Can you work these out from the model? Positions are in its coordinate system, mm. Face numbers are marked on the shaded views. A direction names the side the tool comes from. Round coordinates to 2 decimals unless told otherwise and drop trailing zeros. Loops run counter-clockwise (first coordinate to the right, second up) from the corner with the lowest first, then second, coordinate; pieces in that order, holes last.
(1) If I drill on line 1 along Y through (x, z) = (-0.25, -1.75); line 2 along Y through (x, z) = (0, 3.05); line 3 along Y through (x, z) = (0.25, 4.25), over which ranges is the centre line in solid material (lowest first)?
(2) I want a section at A-A on z = 3.75. Write out the boundary of the cut face in (x, y), plus the area to 3 significant figures.
(3) Will these pins go through, and if not, where does the flat tip stop? pin 1 Ø2 at (x, z) = (3, 0) entering from -Y; pin 2 Ø1 at (y, z) = (3, 1) entering from +X; pin 3 Ø3.5 at (x, y) = (-0.5, 2) entering from -Z.
(4) Thinking about a two-plate mould opening in Y: for the marked faces 3 and 4, which applies, released by +Y, released by -Y, zero draft, split by the parting line, or undercut?
(5) I want a section at B-B on z = 0.5. Write out the boundary of the cut face in (x, y), plus the area to 3 significant figures.
(6) Which directions (+Z, -Z, +X, -X, +Y, -Y) give clear straight access to the entire face, cutting with the end or side of a thin tool? Please do the marked faces 1 and 2.
from build123d import *

# Parameters (mm, degrees)
SKETCH1_R           = 8.5
BOSS_EXTRUDE1_DEPTH = 4.4
SKETCH3_R           = 5.8
CUT_EXTRUDE1_DEPTH  = 4
BOSS_EXTRUDE3_START = 3
SKETCH4_R           = 8.5
SKETCH4_R_2         = 7.5
BOSS_EXTRUDE3_DEPTH = 3
BOSS_EXTRUDE4_DEPTH = 0.6


with BuildPart() as part:
    # Sketch1 → Boss-Extrude1 (new body)
    with BuildSketch(Plane.XY):
        Circle(SKETCH1_R)
    extrude(amount=BOSS_EXTRUDE1_DEPTH)

    # Sketch3 → Cut-Extrude1 (cut)
    with BuildSketch(Plane(origin=(0, 0, 0), x_dir=(-1, 0, 0), z_dir=(0, 0, -1))):
        Circle(SKETCH3_R)
    extrude(amount=-CUT_EXTRUDE1_DEPTH, mode=Mode.SUBTRACT)

    # Sketch4 → Boss-Extrude3 (add)
    with BuildSketch(Plane(origin=(0, 0, 0), x_dir=(-1, 0, 0), z_dir=(0, 0, -1)).offset(BOSS_EXTRUDE3_START)):
        Circle(SKETCH4_R)
        Circle(SKETCH4_R_2, mode=Mode.SUBTRACT)
    extrude(amount=-BOSS_EXTRUDE3_DEPTH)

    # Sketch6 → Cut-Revolve1 (revolve, cut)
    with BuildSketch(Plane(origin=(0, 0, 0), x_dir=(1, 0, 0), z_dir=(0, 1, 0)), mode=Mode.PRIVATE) as cut_revolve1_sk:
        Polygon((7.5, 0), (5.8, -1.7), (5.8, 0), align=None)
    revolve(cut_revolve1_sk.sketch.rotate(Axis((0, 0, -5.5), (0, 0, 1)), 180), axis=Axis((0, 0, -5.5), (0, 0, 1)), mode=Mode.SUBTRACT)

    # Sketch2 → Boss-Extrude4 (add)
    with BuildSketch(Plane.XY.offset(4.4)):
        with BuildLine():
            Line((3.632089791, -3.751482391), (5.223035304, -5.300560917))
            Line((5.223035304, -5.300560917), (1.278724407, -5.300560917))
            Line((1.278724407, -5.300560917), (1.278724407, -1.424559314))
            Line((1.278724407, -1.424559314), (2.845431137, -2.97363784))
            add(Edge.make_bspline(
                [(2.845431137, -2.97363784), (2.95632075, -2.861034584), (3.174405253, -2.639579891), (3.459213248, -2.278430368), (3.70074243, -1.902868481), (3.898794049, -1.512590066), (4.05164193, -1.107607515), (4.159151203, -0.687847174), (4.228166952, -0.253828699), (4.236197805, 0.041257842), (4.240262868, 0.190624981)],
                knots=[0, 0, 0, 0, 1.065567823, 2.095632081, 3.096325677, 4.073630942, 5.042774034, 6.010294195, 6.992849145, 8, 8, 8, 8], degree=3))
            add(Edge.make_bspline(
                [(4.240262868, 0.190624981), (4.236521971, 0.339185131), (4.229157297, 0.631654273), (4.16882099, 1.061635432), (4.066106532, 1.474567413), (3.926128217, 1.87176171), (3.742510622, 2.251822429), (3.522034828, 2.616182439), (3.260511136, 2.964392602), (2.959512286, 3.288301222), (2.634991287, 3.589186758), (2.288400016, 3.852429668), (1.924418043, 4.074704619), (1.543968163, 4.255940011), (1.147484032, 4.397650491), (0.735726783, 4.499431142), (0.30732266, 4.560199144), (0.016301238, 4.567516752), (-0.131532004, 4.571233955)],
                knots=[0, 0, 0, 0, 1.036283767, 2.0401233, 3.022098945, 4.001181535, 4.973115426, 5.961928152, 6.96848522, 8.005845645, 9.043206071, 10.052850644, 11.037284036, 12.013841621, 12.988096842, 13.970072486, 14.968836162, 16, 16, 16, 16], degree=3))
            add(Edge.make_bspline(
                [(-0.131532004, 4.571233955), (-0.280088337, 4.567459865), (-0.573277686, 4.560011356), (-1.00473588, 4.499828874), (-1.418221214, 4.397341401), (-1.816346635, 4.258767128), (-2.196115848, 4.076581392), (-2.560226583, 3.855519569), (-2.903891125, 3.590363046), (-3.230152733, 3.293680989), (-3.527552899, 2.967768525), (-3.790083641, 2.621418652), (-4.007152184, 2.255441675), (-4.192132355, 1.876734755), (-4.328849407, 1.477819774), (-4.432036389, 1.063874926), (-4.49207445, 0.632358672), (-4.499542755, 0.339177282), (-4.503326876, 0.190624981)],
                knots=[0, 0, 0, 0, 1.035427484, 2.043509704, 3.02964574, 4.001383878, 4.977134532, 5.960754486, 6.96548856, 7.998532717, 9.031576874, 10.037302222, 11.022653504, 11.993784286, 12.97035426, 13.956490296, 14.964572516, 16, 16, 16, 16], degree=3))
            add(Edge.make_bspline(
                [(-4.503326876, 0.190624981), (-4.499608767, 0.046452954), (-4.492253992, -0.238733168), (-4.430784866, -0.659467236), (-4.331445734, -1.067569513), (-4.19188491, -1.463967176), (-4.01175723, -1.848290505), (-3.795509518, -2.222691708), (-3.53699416, -2.583569925), (-3.337577276, -2.80718571), (-3.236299632, -2.920753225)],
                knots=[0, 0, 0, 0, 1.00470997, 1.987412856, 2.957385615, 3.929100441, 4.911910053, 5.912278307, 6.939710965, 8, 8, 8, 8], degree=3))
            Line((-3.236299632, -2.920753225), (-4.005330081, -3.691987199))
            add(Edge.make_bspline(
                [(-4.005330081, -3.691987199), (-4.135271474, -3.549666878), (-4.391109201, -3.269456652), (-4.719311464, -2.815225768), (-5.004332233, -2.351060045), (-5.230143754, -1.867949003), (-5.411519251, -1.371567784), (-5.538708635, -0.859768832), (-5.615741653, -0.332482335), (-5.62622625, 0.023633109), (-5.631532004, 0.203846134)],
                knots=[0, 0, 0, 0, 1.067518229, 2.101804739, 3.101067448, 4.082788766, 5.052650977, 6.026360255, 7.001235147, 8, 8, 8, 8], degree=3))
            add(Edge.make_bspline(
                [(-5.631532004, 0.203846134), (-5.627457502, 0.390708619), (-5.619432553, 0.758744313), (-5.538520982, 1.298672582), (-5.414249777, 1.818110739), (-5.235843212, 2.315782791), (-5.011649393, 2.795149888), (-4.73042278, 3.250028561), (-4.403608666, 3.686459458), (-4.028557339, 4.094332656), (-3.619894559, 4.468793147), (-3.185532677, 4.799872374), (-2.726214157, 5.075680655), (-2.248647615, 5.304538365), (-1.749434149, 5.482282496), (-1.22855864, 5.606437585), (-0.687143546, 5.687225777), (-0.318389709, 5.695331626), (-0.131532004, 5.699439083)],
                knots=[0, 0, 0, 0, 1.036548909, 2.041538722, 3.023471865, 3.997074745, 4.970976362, 5.955504589, 6.960097362, 7.993216813, 9.026336264, 10.033383207, 11.019278073, 11.994927594, 12.968530475, 13.95442534, 14.963451091, 16, 16, 16, 16], degree=3))
            add(Edge.make_bspline(
                [(-0.131532004, 5.699439083), (0.054595523, 5.695345882), (0.421895617, 5.687268445), (0.961779629, 5.606175508), (1.481981128, 5.482330381), (1.981120847, 5.30443921), (2.458381777, 5.076303735), (2.916213765, 4.799218389), (3.350458552, 4.468265022), (3.760990035, 4.094356336), (4.138315988, 3.687117495), (4.465256719, 3.250043032), (4.745894958, 2.794580246), (4.973314126, 2.316382013), (5.151012636, 1.818029141), (5.275504478, 1.29869497), (5.356356116, 0.758738455), (5.364389309, 0.390706646), (5.368467996, 0.203846134)],
                knots=[0, 0, 0, 0, 1.032739074, 2.037985287, 3.024131681, 3.997982954, 4.97388139, 5.956539052, 6.96384292, 8.000239142, 9.03637858, 10.041227652, 11.026007058, 12.001905494, 12.975756767, 13.957940427, 14.96318664, 16, 16, 16, 16], degree=3))
            add(Edge.make_bspline(
                [(5.368467996, 0.203846134), (5.363680287, 0.016248292), (5.354227058, -0.354159577), (5.270200799, -0.899409197), (5.132702079, -1.4248242), (4.943051484, -1.932209131), (4.696350305, -2.419026583), (4.396055183, -2.886430144), (4.043519788, -3.336927549), (3.770889078, -3.611628912), (3.632089791, -3.751482391)],
                knots=[0, 0, 0, 0, 1.01247621, 1.999112297, 2.970711092, 3.940884138, 4.91819732, 5.911673186, 6.936809893, 8, 8, 8, 8], degree=3))
        make_face()
    extrude(amount=BOSS_EXTRUDE4_DEPTH)


solid = part.part
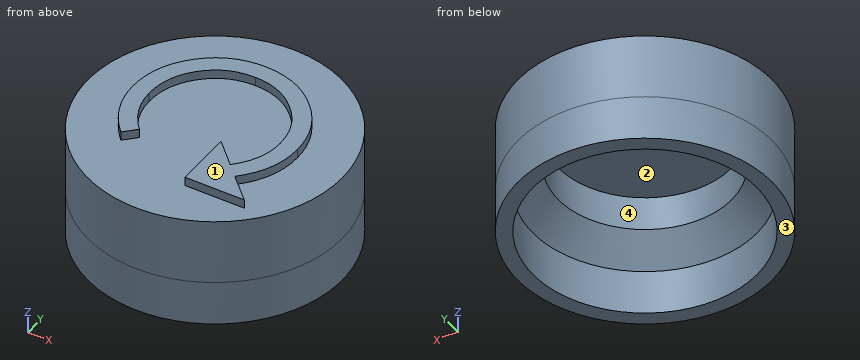
Filled sheet:
1. line 1: y = -8.5 to -7.5, 7.5 to 8.5
1. line 2: y = -8.5 to -5.8, 5.8 to 8.5
1. line 3: y = -8.5 to 8.5
2. outline: circle Ø17 at (0, 0); hole circle Ø11.6 at (0, 0)
2. area: 121 mm2
3. pin 1: stops at y = -8.26
3. pin 2: stops at x = 8.12
3. pin 3: stops at z = 4
4. face 3: zero draft
4. face 4: undercut
5. outline: circle Ø17 at (0, 0); hole circle Ø14 at (0, 0)
5. area: 73.0 mm2
6. face 1: +Z, +X, -X, +Y, -Y
6. face 2: -Z
